Can you work these out from the model? Positions are in its coordinate system, mm. A direction names the side the tool comes from. Round coordinates to 2 decimals unless told otherwise and drop trailing zeros. Order: outer loops, then holes, each group sorted by start corner. A loop starts at its lowest first (then second) coordinate and runs counter-clockwise, first axis right, second up.
from build123d import *

# Parameters (mm, degrees)
SKETCH_1_W          = 150
SKETCH_1_H          = 130
EXTRUDE_1_DEPTH     = 25
SKETCH_2_W          = 150
SKETCH_2_H          = 55
EXTRUDE_2_DEPTH     = 50
SKETCH_4_R          = 8
CUT_EXTRUDE_2_DEPTH = 112.130553854
RIB_1_REACH         = 126.399
SKETCH_5_WALL_W     = 313.297106092
SKETCH_5_WALL_H     = 20
SKETCH_6_W          = 50
SKETCH_6_H          = 35
CUT_EXTRUDE_3_DEPTH = 180.861057486
SKETCH_8_W          = 13
SKETCH_8_H          = 55
CUT_EXTRUDE_4_DEPTH = 15


with BuildPart() as part:
    # Эскиз1 → Бобышка-Вытянуть1 (new body)
    with BuildSketch(Plane.XY):
        Rectangle(SKETCH_1_W, SKETCH_1_H)
    extrude(amount=EXTRUDE_1_DEPTH)

    # Эскиз2 → Бобышка-Вытянуть2 (add)
    with BuildSketch(Plane.XY.offset(25)):
        Rectangle(SKETCH_2_W, SKETCH_2_H)
    extrude(amount=EXTRUDE_2_DEPTH)

    # Эскиз4 → Вырез-Вытянуть2 (cut, through all)
    with BuildSketch(Plane.XY.offset(25)):
        with Locations((45, -50)):
            Circle(SKETCH_4_R)
    cut_extrude_2 = extrude(amount=-CUT_EXTRUDE_2_DEPTH, mode=Mode.SUBTRACT)

    # Эскиз5 wall → Ребро1 (add, up to next)
    with BuildSketch(Plane(origin=(0, -46.25, 50), x_dir=(0, -0.6, -0.8), z_dir=(0, 0.8, -0.6)), mode=Mode.PRIVATE) as rib_1_sk1:
        Rectangle(SKETCH_5_WALL_W, SKETCH_5_WALL_H)
    rib_1_tool1 = extrude(rib_1_sk1.sketch, amount=RIB_1_REACH, mode=Mode.PRIVATE) - part.part
    add(rib_1_tool1.solids().sort_by_distance((0, -46.25, 50))[0])

    # Зеркальное отражение1: Вырез-Вытянуть2 across plane
    add(cut_extrude_2.mirror(Plane(origin=(0, 0, 0), x_dir=(0, 0, 1), z_dir=(1, 0, 0))), mode=Mode.SUBTRACT)

    # Эскиз6 → Вырез-Вытянуть3 (cut, through all)
    with BuildSketch(Plane(origin=(75, 0, 0), x_dir=(0, 0, -1), z_dir=(1, 0, 0))):
        with Locations((-37, 0)):
            Rectangle(SKETCH_6_W, SKETCH_6_H)
    extrude(amount=-CUT_EXTRUDE_3_DEPTH, mode=Mode.SUBTRACT)

    # Эскиз8 → Вырез-Вытянуть4 (cut)
    with BuildSketch(Plane(origin=(75, 0, 0), x_dir=(0, 0, -1), z_dir=(1, 0, 0))):
        with Locations((-55.5, 0)):
            Rectangle(SKETCH_8_W, SKETCH_8_H)
    cut_extrude_4 = extrude(amount=-CUT_EXTRUDE_4_DEPTH, mode=Mode.SUBTRACT)

    # Зеркальное отражение2: Вырез-Вытянуть4 across plane
    add(cut_extrude_4.mirror(Plane(origin=(0, 0, 0), x_dir=(0, 0, 1), z_dir=(1, 0, 0))), mode=Mode.SUBTRACT)


solid = part.part
(1) If we mould it in two halves opening along Y, with no side actions, what happens to faces 5 (the face through (1, 0, 12)), 6 (the face through (-43, -27.5, 50)), 7 (the face through (-68, 22, 49))? For each: pulls with the +Y half, pulls with the -Y half, needs draft (parallel to the pull), parting line crosses it, or undercut.
(2) I want a section at D-D, the plane z = 14. List the corners of the cut face in (x, y) for me, plus the area to 3 significant figures.
(3) On a 3-axis mill with a long thin cutter (end or side, diameter ignored), from which of +Z, -Z, +X, -X, +Y, -Y can I reach the whole of each face in a straight line? I mean faces 1 (the face through (-43, -42, 25)), 2 (the face through (1, 17.5, 37)), 3 (the face through (42, -27.5, 50)), 4 (the face through (-68, -23, 49)). Say none if no direction works.
(4) I want a section at C-C, the plane y = 5. List the corners of the cut face in (x, z) for me.
(5) I want a section at B-B, the plane z = 53. List the corners of the cut face in (x, y) for me.
(6) Please list where these lines run through material, in increasing order: probe 1 along Y at (x, z) = (45, 18); probe 2 along Y at (x, z) = (-45, 8); probe 3 along Y at (x, z) = (-49.5, 20).
(7) I want a section at A-A, the plane x = 45. List the corners of the cut face in (y, z) for me, plus the area to 3 significant figures.
(8) I'm going to push flat-ended pins straight in: pin 1 Ø25 at (x, z) = (21, 25.5) entering from +Y; pin 2 Ø4 at (y, z) = (-34, 63) entering from -X; pin 3 Ø5 at (y, z) = (-23, 56.5) entering from -X; pin 4 Ø15 at (x, z) = (-1, 37) entering from -Y (3 decimals). Where does each tip first touch, or does it pass through?
Ans:
1. face 5: undercut
1. face 6: pulls with the -Y half
1. face 7: needs draft
2. outline: (-75, -65) - (75, -65) - (75, -17.5) - (-75, -17.5) - close; (-75, 17.5) - (75, 17.5) - (75, 65) - (-75, 65) - close; hole circle Ø16 at (-45, -50); hole circle Ø16 at (45, -50)
2. area: 13,800 mm2
3. face 1: +Z, -X, -Y
3. face 2: +X, -X
3. face 3: +Z, +X, -Y
3. face 4: -X, +Y, -Y
4. outline: (-75, 0) - (75, 0) - (75, 12) - (-75, 12) - close; (-75, 62) - (75, 62) - (75, 75) - (-75, 75) - close
5. outline: (-60, -27.5) - (-10, -27.5) - (-10, -44) - (10, -44) - (10, -27.5) - (60, -27.5) - (60, -17.5) - (-60, -17.5) - close; (-60, 17.5) - (60, 17.5) - (60, 27.5) - (-60, 27.5) - close
6. probe 1: y = -65 to -58, -42 to -17.5, 17.5 to 65
6. probe 2: y = -65 to -58, -42 to 65
6. probe 3: y = -65 to -56.61, -43.39 to -17.5, 17.5 to 65
7. outline: (-65, 0) - (-58, 0) - (-58, 25) - (-65, 25) - close; (-42, 0) - (65, 0) - (65, 25) - (27.5, 25) - (27.5, 75) - (-27.5, 75) - (-27.5, 25) - (-42, 25) - close; hole (-17.5, 12) - (17.5, 12) - (17.5, 62) - (-17.5, 62) - close
7. area: 3,850 mm2
8. pin 1: stops at y = 65
8. pin 2: stops at x = -10
8. pin 3: stops at x = -60
8. pin 4: stops at y = -61.625
